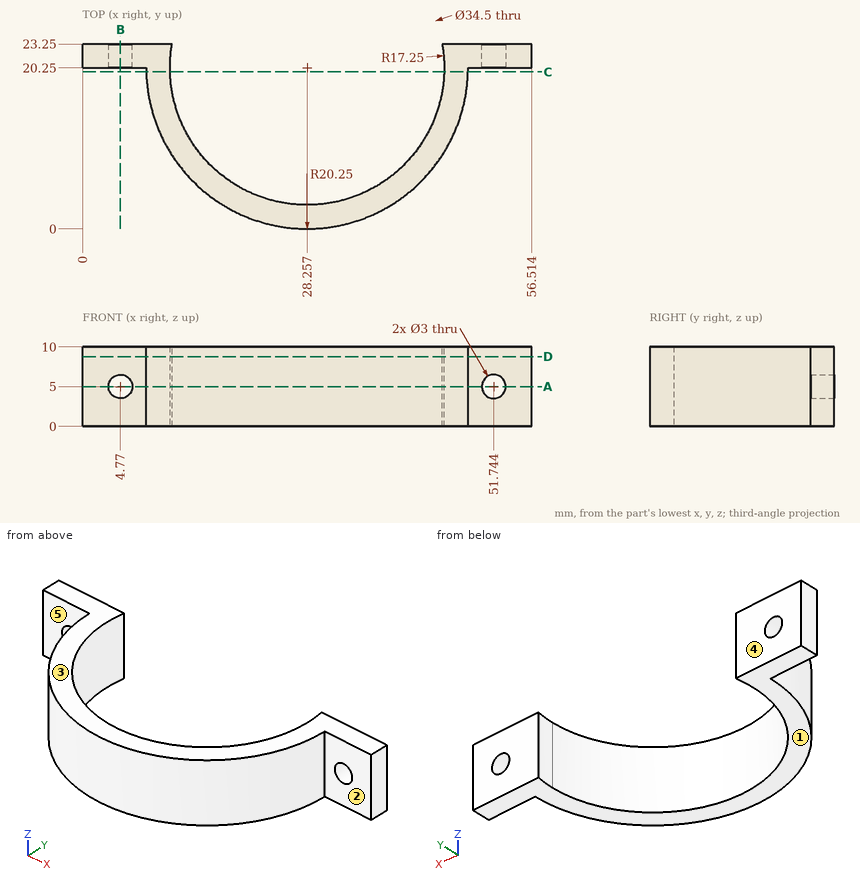
Input: dimensioned drawing with shaded views. Units: mm. Origin: part minimum x, y, z. A direction names the side the tool comes from. Give positions to 0.01 mm unless a question says otherwise; leave off trailing zeros. Order: outer loops, then holes, each group sorted by start corner. A loop starts at its lowest first (then second) coordinate and runs counter-clockwise, first axis right, second up. Notation, with made-up numbers: (55, -26.5) -> (102, -26.5) arc R13 ccw to (102, -16.5) -> close; hole circle Ø11 at (53, -25). An arc over 180 degrees is marked (long way). Answer as a JSON object with one key per item and string values.
Q1. Draft query along Z for the marked faces 1, 2 and 3. Return one class per face: released by +Z, released by -Z, zero draft, split by the parting line, or undercut.
Entries:
{"face 1": "released by -Z", "face 2": "zero draft", "face 3": "released by +Z"}
Q2. Section D-D (z = 8.75). Output: boundary loops of the cut face in (x, y), plus the area to 3 significant figures.
Entries:
{"outline": "(0, 20.25) -> (8.01, 20.25) arc R20.25 ccw to (48.51, 20.25) -> (56.51, 20.25) -> (56.51, 23.25) -> (45.24, 23.25) arc R17.25 cw (long way) to (11.27, 23.25) -> (0, 23.25) -> close", "area": "243 mm^2"}
Q3. Material intervals for probe 1 along Z at (x, y) = (4.77, 21.7); probe 2 along Y at (x, z) = (53.5, 2.75); probe 3 along X at (y, z) = (7.5, 6.25) (1 decimal), sorted ascending.
Entries:
{"probe 1": "z = 0 to 3.5, 6.5 to 10", "probe 2": "y = 20.25 to 23.25", "probe 3": "x = 12.5 to 16.6, 39.9 to 44"}
Q4. Section B-B (x = 4.77). Output: boundary loops of the cut face in (y, z), plus the area to 3 significant figures.
Entries:
{"outline": "(20.25, 0) -> (23.25, 0) -> (23.25, 3.5) -> (20.25, 3.5) -> close; (20.25, 6.5) -> (23.25, 6.5) -> (23.25, 10) -> (20.25, 10) -> close", "area": "21.0 mm^2"}
Q5. Access query for the marked faces 4 and 5. Directions: +Z, -Z, +X, -X, +Y, -Y. A direction counts if a zero-diameter tool reaches every point of the face in a straight line with its end or side. Return the directions, or none.
Entries:
{"face 4": "+Z, -Z, +X, -X, +Y", "face 5": "+Z, -Z, -X, -Y"}
Q6. Section A-A (z = 5). Output: boundary loops of the cut face in (x, y), plus the area to 3 significant figures.
Entries:
{"outline": "(0, 20.25) -> (3.27, 20.25) -> (3.27, 23.25) -> (0, 23.25) -> close; (6.27, 20.25) -> (8.01, 20.25) arc R20.25 ccw to (48.51, 20.25) -> (50.24, 20.25) -> (50.24, 23.25) -> (45.24, 23.25) arc R17.25 cw (long way) to (11.27, 23.25) -> (6.27, 23.25) -> close; (53.24, 20.25) -> (56.51, 20.25) -> (56.51, 23.25) -> (53.24, 23.25) -> close", "area": "225 mm^2"}
Q7. First-contact query: pin 1 (2.5 mm diameter, centred on x = 52, z = 6.5, fed in from -Y); pin 2 (2.5 mm diameter, centred on x = 4.77, z = 5, fed in from +Y); pin 3 (6 mm diameter, centred on y = 16, z = 7.5, fed in from -X); pin 4 (2 mm diameter, centred on x = 43, z = 1, fed in from +Y). Flat tips, straight axial feed; report the tip coordinate or a pass-through.
Entries:
{"pin 1": "stops at y = 20.25", "pin 2": "passes through", "pin 3": "stops at x = 8.05", "pin 4": "stops at y = 13.2"}
Q8. Section C-C (y = 19.75). Output: boundary loops of the cut face in (x, z), plus the area to 3 significant figures.
Entries:
{"outline": "(8.01, 0) -> (11.01, 0) -> (11.01, 10) -> (8.01, 10) -> close; (45.5, 0) -> (48.5, 0) -> (48.5, 10) -> (45.5, 10) -> close", "area": "60.0 mm^2"}
